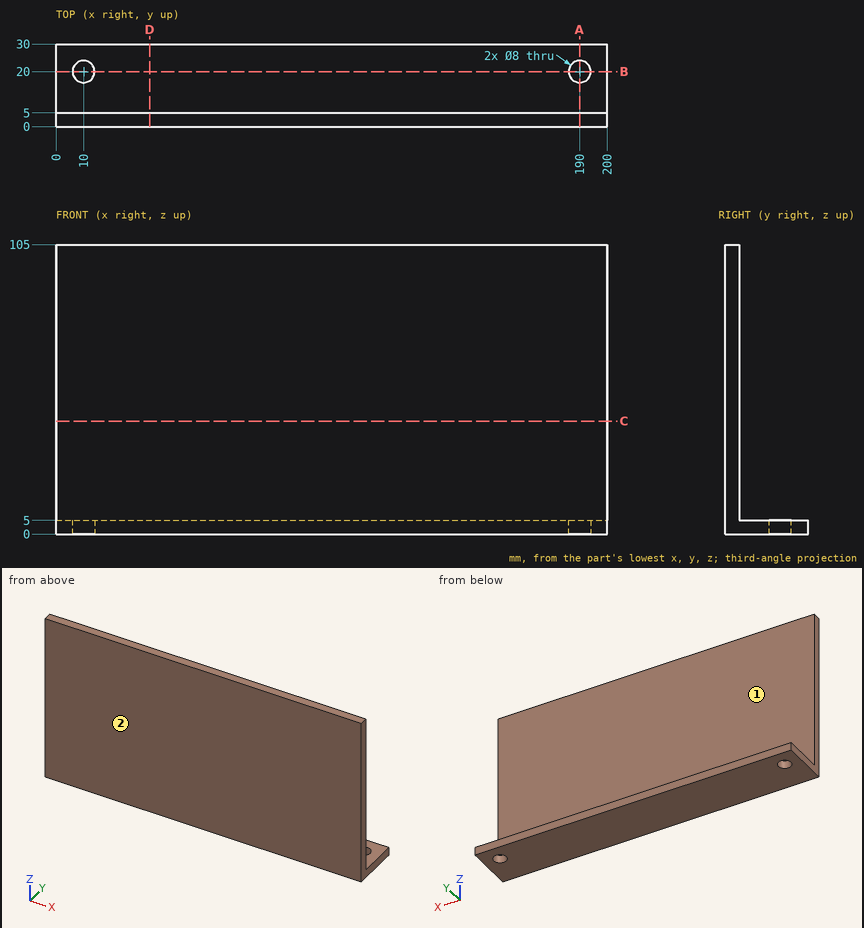
Print and shaded views of the part. All mm, measured from the part's lowest x, y and z. A direction names the side the tool comes from. Round coordinates to 2 decimals unless told otherwise and drop trailing zeros. Write each loop counter-clockwise with the first axis right and the second up, starting at its lowest first coordinate (ties: lowest second). Pieces come first, ordered by that corner, then holes.
(1) 3-axis set-ups, long thin cutter, end or side, ignore diameter. For the marked faces 1 and 2: which of +Z, -Z, +X, -X, +Y, -Y reach the whole face in a straight line?
(2) Probe line 1 along Y through (x, z) = (10, 1); line 2 along Y through (x, z) = (164, 70). List the from-to ranges inside material, lowest first.
(3) Drop flat-ended pins along their axis: P1, Ø3, axis at x = 123, z = 22, coming from the +Y side; P2, Ø13, axis at x = 10, y = 20, coming from the +Z side; P3, Ø6, axis at y = 9.5, z = 30, coming from the -X side. Give the stop position or say it passes through.
(4) Slice it at B-B, the plane y = 20. Write the cut outline in (x, z).
(5) Slice it at A-A, the plane x = 190. Write the cut outline in (y, z), and give its area (3 significant figures).
(6) Slice it at C-C, the plane z = 41. Write the cut outline in (x, y), and give its area (3 significant figures).
(7) Slice it at D-D, the plane x = 34. Write the cut outline in (y, z), and give its area (3 significant figures).
From the geometry:
1. face 1: +Z, +X, -X, +Y
1. face 2: +Z, -Z, +X, -X, -Y
2. line 1: y = 0 to 16, 24 to 30
2. line 2: y = 0 to 5
3. P1: stops at y = 5
3. P2: stops at z = 5
3. P3: passes through
4. outline: (0, 0) - (6, 0) - (6, 5) - (0, 5) - close; (14, 0) - (186, 0) - (186, 5) - (14, 5) - close; (194, 0) - (200, 0) - (200, 5) - (194, 5) - close
5. outline: (0, 0) - (16, 0) - (16, 5) - (5, 5) - (5, 105) - (0, 105) - close; (24, 0) - (30, 0) - (30, 5) - (24, 5) - close
5. area: 610 mm2
6. outline: (0, 0) - (200, 0) - (200, 5) - (0, 5) - close
6. area: 1,000 mm2
7. outline: (0, 0) - (30, 0) - (30, 5) - (5, 5) - (5, 105) - (0, 105) - close
7. area: 650 mm2
